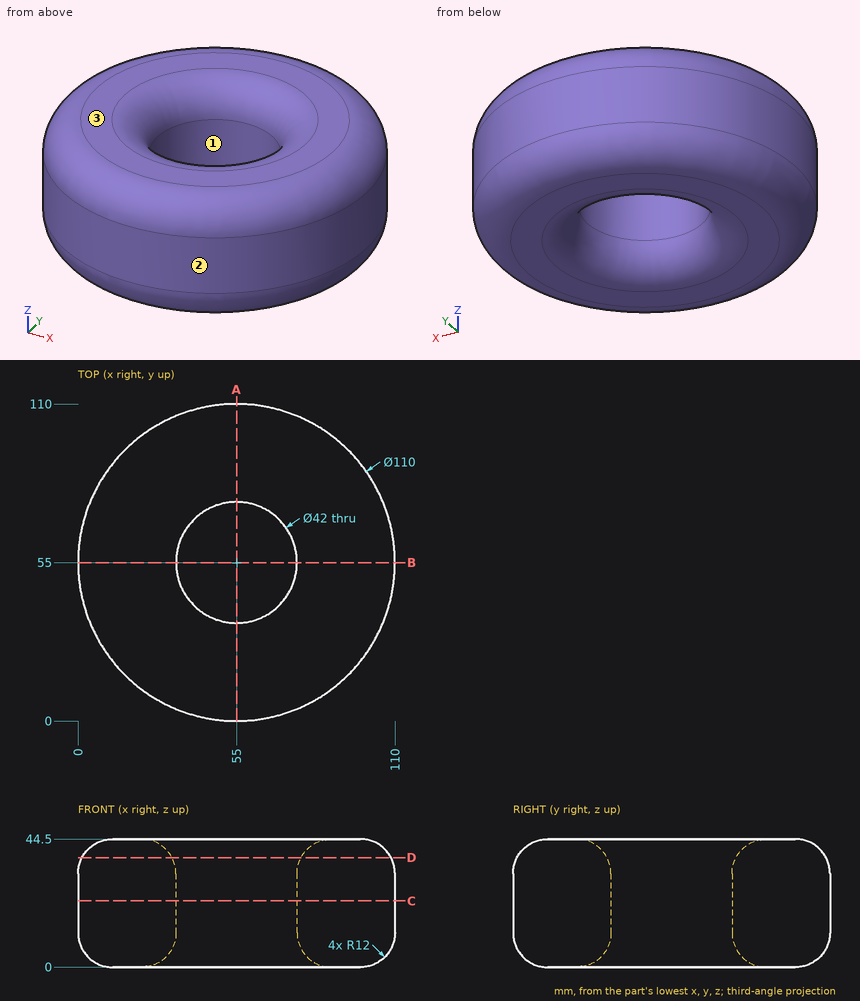
Could you check a few things on this drawing? It's one solid part, dimensions in mm from its lowest x, y, z. Coordinates: 2 decimals unless noted, no trailing zeros. Order: outer loops, then holes, each group sorted by start corner. A loop starts at its lowest first (then second) coordinate and runs counter-clockwise, first axis right, second up. Notation, with made-up numbers: M 71,32.5 L 108,32.5 A9 cw 108,48.5 Z; hole C 27,50.5 d5. An arc over 180 degrees is marked long. Answer as a JSON object with one key per item and string values. Group by question number.
(1) Suppose I cut it at A-A, the plane x = 55. Please give me the cut outline in (y, z).
(2) For pin 1 (1.5 mm diameter, centred on y = 22.5, z = 24.5, fed in from +X); pin 2 (25 mm diameter, centred on x = 55, y = 55, fed in from +Z); pin 3 (10 mm diameter, centred on x = 96.5, z = 23.5, fed in from -Y); pin 4 (2 mm diameter, centred on y = 90.5, z = 36, fed in from -X), each with a flat end and sliding along its axis, tell me the tip position at first contact or that it passes through.
(3) If we mould it in two halves opening along X, with no side actions, what happens to the marked faces 1, 2 and 3? For each: released by +X, released by -X, zero draft, split by the parting line, or undercut.
(4) I need wall thicknesses on probe 1 along Y at (x, z) = (55, 27); probe 2 along X at (y, z) = (61, 19.5); probe 3 along X at (y, z) = (44.5, 28.5). Which ranges of each line are inside material? Lowest first, please.
(5) Suppose I cut it at D-D, the plane z = 38. Please give me the cut outline in (x, y), then the cut area to 3 significant figures.
(6) Suppose I cut it at C-C, the plane z = 23. Please give me the cut outline in (x, y), then the cut area to 3 significant figures.
Values found:
{
 "1": {"outline": "M 0,12 A12 ccw 12,0 L 22,0 A12 ccw 34,12 L 34,32.5 A12 ccw 22,44.5 L 12,44.5 A12 ccw 0,32.5 Z; M 76,12 A12 ccw 88,0 L 98,0 A12 ccw 110,12 L 110,32.5 A12 ccw 98,44.5 L 88,44.5 A12 ccw 76,32.5 Z"},
 "2": {"pin 1": "stops at x = 99.91", "pin 2": "passes through", "pin 3": "stops at y = 13.86", "pin 4": "stops at x = 12.76"},
 "3": {"face 1": "undercut", "face 2": "split by the parting line", "face 3": "zero draft"},
 "4": {"probe 1": "y = 0 to 34, 76 to 110", "probe 2": "x = 0.33 to 34.88, 75.12 to 109.67", "probe 3": "x = 1.01 to 36.81, 73.19 to 108.99"},
 "5": {"outline": "C 55,55 d107.33; hole C 55,55 d44.67", "area": "7,480 mm^2"},
 "6": {"outline": "C 55,55 d110; hole C 55,55 d42", "area": "8,120 mm^2"}
}
